Verification items for the finished model (mm, model axes). Face numbers are marked on the shaded views. A direction names the side the tool comes from. Coordinates: 2 decimals unless noted, no trailing zeros. Loops run counter-clockwise (first coordinate to the right, second up) from the corner with the lowest first, then second, coordinate; pieces in that order, holes last. Notation, with made-up numbers: (24.25, 4.5) - (42.25, 4.5) arc R18 ccw to (42.25, 20.5) - close; hole circle Ø9 at (60, -8). An arc over 180 degrees is marked (long way). One line per item, written item: value. Start each with the question number.
(1) Section check B-B (x = 20). Count the separate pieces of the cut face and the enclosed holes in it, plus the area to 3 significant figures.
(2) Section check D-D (y = 11). Record the boundary of the cut face in (x, z) (3 decimals).
(3) Section check C-C (z = 20.5). Record the boundary of the cut face in (x, y), plus the area to 3 significant figures.
(4) Set-up check for the marked faces 5, 6 and 7: record each of +Z, -Z, +X, -X, +Y, -Y from which the full face is reachable in a straight line by a thin tool's end or side.
(5) Thickness scan on probe 1 along Y at (x, z) = (13.5, 31.5); probe 2 along Y at (x, z) = (39.5, 13); probe 3 along Z at (x, y) = (64.5, 0). Record the ranges inside material, lowest first. Write a range as [from, to].
(6) Section check A-A (x = 40). Record the boundary of the cut face in (y, z), plus the area to 3 significant figures.
(7) Gauge pin test, flat ends, axial feed: P1, Ø6.5, axis at y = 9.5, z = 13.5, coming from the +X side; P2, Ø2, axis at x = 66.5, z = 12.5, coming from the +Y side; P3, Ø2, axis at x = 72, z = 9, coming from the -Y side; P4, Ø4.5, axis at x = 59, z = 16.5, coming from the +Y side. Record the tip position at first contact, or that the pin passes through.
(8) Draft check along X on the marked faces 1, 2, 3 and 4. Enter one of: +X half, -X half, draft (parallel to the pull), parting line (faces both ways), or undercut.
Autodesk Inventor part; units mm, degrees
ref_plane "YZ Plane" through (0, 0, 0) normal (1, 0, 0) x (0, 1, 0)
ref_plane "XZ Plane" through (0, 0, 0) normal (0, 1, 0) x (-1, 0, 0)
ref_plane "XY Plane" through (0, 0, 0) normal (0, 0, 1) x (1, 0, 0)
sketch "Sketch1" plane through (0, 0, 0) normal (0, 0, 1) x (1, 0, 0)
  line L0 (0, 14) -> (52.5, 14)
  line L1 (52.5, 14) -> (52.5, 5.75)
  line L2 (52.5, 5.75) -> (82.5, 5.75)
  line L3 (82.5, 5.75) -> (82.5, -5.75)
  line L4 (82.5, -5.75) -> (52.5, -5.75)
  line L5 (52.5, -5.75) -> (52.5, -14)
  line L6 (52.5, -14) -> (0, -14)
  arc A0 (0, 14) -> (0, -14) centre (0, 0) ccw
  dimension "d0" = 82.5
  dimension "d1" = 30
  dimension "d2" = 14
  dimension "d3" = 11.5
extrude "Extrusion1" add sketch "Sketch1" along normal blind 33
sketch "Sketch2" plane through (0, 0, 0) normal (0, 0, -1) x (-1, 0, 0)
  arc A0 (0, -14) -> (0, 14) centre (0, 0) ccw
  circle A1 centre (0, 0) radius 6
  circle A2 centre (-40, 0) radius 6
  dimension "d6" = 12
  dimension "d8" = 40
extrude "Extrusion2" cut sketch "Sketch2" against normal through all
sketch "Sketch3" plane through (52.5, -5.75, 0) normal (0, -1, 0) x (1, 0, 0)
  line L0 (30, 0) -> (30, 33)
  line L1 (0, 0) -> (0, 33)
  line L2 (25, 18.25) -> (22, 18.25)
  arc A0 (22, 18.25) -> (22, 14.75) centre (22, 16.5) ccw
  line L3 (22, 14.75) -> (25, 14.75)
  arc A1 (25, 14.75) -> (25, 18.25) centre (25, 16.5) ccw
  point P0 (-52.5, 0)
  point P1 (30, 16.5)
  dimension "d11" = 3
  dimension "d13" = 5
  dimension "d14" = 1.75
extrude "Extrusion3" cut sketch "Sketch3" against normal through all
sketch "Sketch4" plane through (52.5, -5.75, 0) normal (0, -1, 0) x (1, 0, 0)
  line L0 (0, 0) -> (0, 33)
  line L1 (5, 8.5) -> (5, 16.5) construction
  line L2 (5, 16.5) -> (5, 24.5) construction
  line L3 (12, 28.5) -> (12, 20.5) construction
  line L4 (12, 20.5) -> (12, 12.5) construction
  line L5 (12, 12.5) -> (12, 4.5) construction
  circle A0 centre (5, 8.5) radius 1.75 construction
  circle A1 centre (5, 16.5) radius 1.75 construction
  circle A2 centre (5, 24.5) radius 1.75 construction
  circle A3 centre (12, 28.5) radius 1.75
  circle A4 centre (12, 20.5) radius 1.75 construction
  circle A5 centre (12, 12.5) radius 1.75 construction
  circle A6 centre (12, 4.5) radius 1.75 construction
  line L6 (0, 0) -> (0, 33)
  circle A7 centre (5.5, 24.5) radius 1.75
  circle A8 centre (13, 20.5) radius 1.75
  circle A9 centre (6.5, 16.5) radius 1.75
  circle A10 centre (14, 12.5) radius 1.75
  circle A11 centre (7.5, 8.5) radius 1.75
  circle A12 centre (15, 4.5) radius 1.75
  point P0 (-52.5, 0)
  point P1 (12, 16.5)
  point P2 (0, 16.5)
  dimension "d17" = 5
  dimension "d18" = 7
  dimension "d19" = 3.5
  dimension "d20" = 8
  dimension "d21" = 0.5
  dimension "d22" = 1
  dimension "d23" = 1.5
  dimension "d24" = 2
  dimension "d25" = 2.5
  dimension "d26" = 3
extrude "Extrusion4" cut sketch "Sketch4" against normal through all
sketch "Sketch5" plane through (0, -14, 0) normal (0, -1, 0) x (1, 0, 0)
  line L0 (52.5, 0) -> (0, 0)
  line L1 (0, 33) -> (52.5, 33)
  line L2 (0, 0) -> (0, 33)
  line L3 (43, -22.7639) -> (43, 127.2361)
  line L4 (37, -22.7639) -> (37, 127.2361)
  line L5 (37, 33) -> (43, 33)
  line L6 (40, 33) -> (40, 0)
  line L7 (0, 14.9) -> (40, 14.9)
  line L8 (20, 14.9) -> (20, 22.275)
  circle A0 centre (20, 22.275) radius 2.75
  line L9 (20, 14.9) -> (20, 7.525)
  circle A1 centre (20, 7.525) radius 2.75
  dimension "d32" = 18.1
  dimension "d34" = 7.375
  dimension "d35" = 5.5
extrude "Extrusion5" cut sketch "Sketch5" against normal through all contours A1 | A0
sketch "Sketch6" plane through (0, 14, 0) normal (0, 1, 0) x (1, 0, 0)
  circle A0 centre (20, -22.275) radius 2.75
  line L0 (22.3094, -18.275) -> (24.6188, -22.275)
  line L1 (24.6188, -22.275) -> (22.3094, -26.275)
  line L2 (22.3094, -26.275) -> (17.6906, -26.275)
  line L3 (17.6906, -26.275) -> (15.3812, -22.275)
  line L4 (15.3812, -22.275) -> (17.6906, -18.275)
  line L5 (17.6906, -18.275) -> (22.3094, -18.275)
  dimension "d38" = 8
extrude "Extrusion6" cut sketch "Sketch6" against normal blind 5
sketch "Sketch7" plane through (0, -14, 0) normal (0, -1, 0) x (1, 0, 0)
  circle A0 centre (20, 7.525) radius 2.75
  line L0 (17.6906, 11.525) -> (22.3094, 11.525)
  line L1 (22.3094, 11.525) -> (24.6188, 7.525)
  line L2 (24.6188, 7.525) -> (22.3094, 3.525)
  line L3 (22.3094, 3.525) -> (17.6906, 3.525)
  line L4 (17.6906, 3.525) -> (15.3812, 7.525)
  line L5 (15.3812, 7.525) -> (17.6906, 11.525)
  dimension "d41" = 8
extrude "Extrusion7" cut sketch "Sketch7" against normal blind 5
sketch "Sketch8" plane through (0, 0, 33) normal (0, 0, 1) x (1, 0, 0)
  circle A0 centre (0, 0) radius 6
  circle A1 centre (40, 0) radius 6
  line L0 (0, 1.5) -> (40, 1.5)
  line L1 (40, 1.5) -> (40, -1.5)
  line L2 (40, -1.5) -> (0, -1.5)
  line L3 (0, -1.5) -> (0, 1.5)
  dimension "d44" = 3
extrude "Extrusion8" cut sketch "Sketch8" against normal through all contours A0 L2 L3 L0 | A0 L0 A1 L2 | L0 L1 L2 A1 picked at (2, 0) picked at (38.0071, -0.1683)
properties part number "distal arm end"
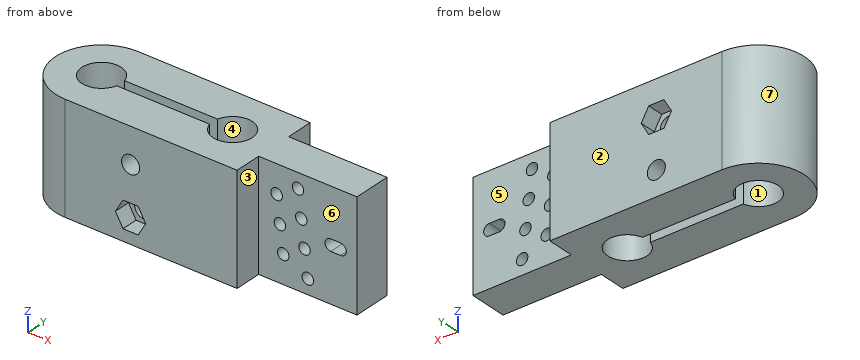
Responses:
1. separate pieces: 6
1. enclosed holes: 0
1. area: 525 mm²
2. outline: (-8.66, 0) - (52.5, 0) - (52.5, 33) - (-8.66, 33) - close; hole (15.381, 22.275) - (17.691, 18.275) - (22.309, 18.275) - (24.619, 22.275) - (22.309, 26.275) - (17.691, 26.275) - close; hole circle Ø5.5 at (20, 7.525)
3. outline: (0, -14) - (17.9, -14) - (17.9, -1.5) - (5.81, -1.5) arc R6 cw (long way) to (5.81, 1.5) - (17.9, 1.5) - (17.9, 9) - (16.41, 9) - (16.41, 14) - (0, 14) arc R14 ccw to start; (22.1, -14) - (52.5, -14) - (52.5, -5.75) - (63.75, -5.75) - (63.75, 5.75) - (52.5, 5.75) - (52.5, 14) - (23.59, 14) - (23.59, 9) - (22.1, 9) - (22.1, 1.5) - (34.19, 1.5) arc R6 cw (long way) to (34.19, -1.5) - (22.1, -1.5) - close; (67.25, -5.75) - (82.5, -5.75) - (82.5, 5.75) - (67.25, 5.75) - close
3. area: 1,650 mm²
4. face 5: +Z, -Z, +X, +Y
4. face 6: +Z, -Z, +X, -Y
4. face 7: +Z, -Z, -X
5. probe 1: y = [-14, -1.5], [1.5, 14]
5. probe 2: y = [-14, -5.98], [5.98, 14]
5. probe 3: z = [0, 19.06], [21.94, 26.75], [30.25, 33]
6. outline: (-14, 0) - (-6, 0) - (-6, 33) - (-14, 33) - close; (6, 0) - (14, 0) - (14, 33) - (6, 33) - close
6. area: 528 mm²
7. P1: stops at x = 52.5
7. P2: passes through
7. P3: stops at y = -5.75
7. P4: stops at y = 5.75
8. face 1: undercut
8. face 2: draft
8. face 3: +X half
8. face 4: undercut
